Part model, mm, in its own coordinate system. Face numbers are marked on the shaded views. A direction names the side the tool comes from. Coordinates: 2 decimals unless noted, no trailing zeros. Order: outer loops, then holes, each group sorted by start corner. A loop starts at its lowest first (then second) coordinate and runs counter-clockwise, first axis right, second up.
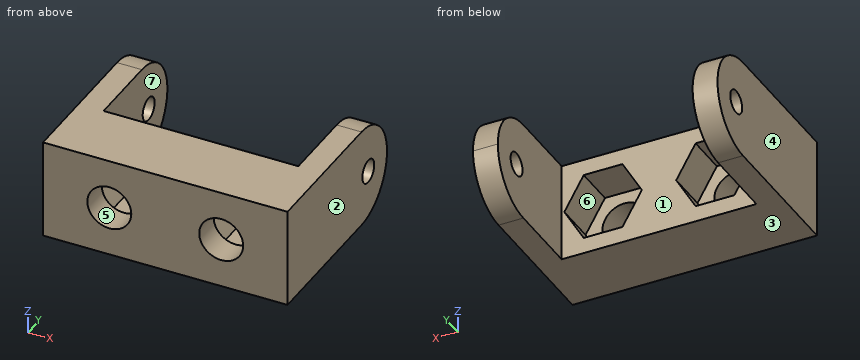
```python
from build123d import *

# Parameters (mm, degrees)
SKETCH_1_W          = 29.5
SKETCH_1_H          = 12
EXTRUDE_1_DEPTH     = 23.4
SKETCH_3_W          = 23.5
SKETCH_3_H          = 12
CUT_EXTRUDE_1_DEPTH = 15
SKETCH_4_R          = 1.4
CUT_EXTRUDE_2_DEPTH = 39.12886046
FILLET_1_RADIUS     = 6
FILLET_1_LENGTH     = 3
MIRROR_START        = 11.75
MIRROR_1_DEPTH      = 3
HOLE_WIZARD_M5_1_D  = 5.3
CUT_EXTRUDE_4_DEPTH = 5


# Read off the part's stored shape, not the designer's step: 镜向1
with BuildPart() as part:
    # 草图1 → 凸台-拉伸1 (new body)
    with BuildSketch(Plane(origin=(0, 0, 0), x_dir=(1, 0, 0), z_dir=(0, 1, 0))):
        Rectangle(SKETCH_1_W, SKETCH_1_H)
    extrude(amount=EXTRUDE_1_DEPTH)

    # 草图3 → 切除-拉伸1 (cut)
    with BuildSketch(Plane(origin=(0, 23.4, 0), x_dir=(1, 0, 0), z_dir=(0, 1, 0))):
        Rectangle(SKETCH_3_W, SKETCH_3_H)
    extrude(amount=-CUT_EXTRUDE_1_DEPTH, mode=Mode.SUBTRACT)

    # 草图4 → 切除-拉伸2 (cut, through all)
    with BuildSketch(Plane.ZY.offset(14.75)):
        with Locations((0, 19)):
            Circle(SKETCH_4_R)
    extrude(amount=-CUT_EXTRUDE_2_DEPTH, mode=Mode.SUBTRACT)

    # 圆角1: full round fillet: the end face becomes a half cylinder, R = half its width
    fillet_1_face = Plane((-13.25, 23.4, 0), x_dir=(-1, 0, 0), z_dir=(0, 1, 0))  # on the end face: x along it, z out of the body
    fillet_1_slab = fillet_1_face.offset(-FILLET_1_RADIUS / 2) * Box(FILLET_1_LENGTH, 2 * FILLET_1_RADIUS, FILLET_1_RADIUS, mode=Mode.PRIVATE)  # the body's end, R deep
    fillet_1_round = Plane((-13.25, 17.4, 0), x_dir=(0, 1, 0), z_dir=(-1, 0, 0)) * Cylinder(FILLET_1_RADIUS, FILLET_1_LENGTH, mode=Mode.PRIVATE)  # its axis R under the face
    add(fillet_1_slab - fillet_1_round, mode=Mode.SUBTRACT)

    # 镜向1 outline → 镜向1 (cut)
    with BuildSketch(Plane.YZ.offset(MIRROR_START)):
        with BuildLine():
            Line((23.4, 6), (17.4, 6))
            ThreePointArc((17.4, 6), (21.642640687, 4.242640687), (23.4, 0))
            Line((23.4, 0), (23.4, 6))
        make_face()
        with BuildLine():
            Line((23.4, -6), (23.4, 0))
            ThreePointArc((23.4, 0), (21.642640687, -4.242640687), (17.4, -6))
            Line((17.4, -6), (23.4, -6))
        make_face()
    extrude(amount=MIRROR_1_DEPTH, mode=Mode.SUBTRACT)

    # M5 间隙孔1 (through all)
    with Locations(Plane(origin=(0, 0, 0), x_dir=(-1, 0, 0), z_dir=(0, -1, 0))):
        with Locations((-6.75, 0), (6.75, 0)):
            Hole(HOLE_WIZARD_M5_1_D / 2)

    # 草图10 → 切除-拉伸4 (cut)
    with BuildSketch(Plane.XZ.offset(-8.4)):
        Polygon((2.07346282, 0), (4.41173141, -4.05), (9.08826859, -4.05), (11.42653718, 0), (9.08826859, 4.05), (4.41173141, 4.05), align=None)
        Polygon((-11.42653718, 0), (-9.08826859, -4.05), (-4.41173141, -4.05), (-2.07346282, 0), (-4.41173141, 4.05), (-9.08826859, 4.05), align=None)
    extrude(amount=CUT_EXTRUDE_4_DEPTH, mode=Mode.SUBTRACT)


solid = part.part
```
(1) Pull direction X, two halves, no side cores. Call the marked faces 1, 2, 3 and 4: +X half, -X half, draft (parallel to the pull), parting line (faces both ways), or undercut.
(2) Drop flat-ended pins along their axis: pin 1 (6.5 mm diameter, centred on x = -5.5, z = -2, fed in from +Y); pin 2 (3 mm diameter, centred on x = 6.75, z = 0, fed in from -Y); pin 3 (6 mm diameter, centred on x = -6.75, z = 0, fed in from +Y). Give the stop position or say it passes through.
(3) Probe line 1 (X direction, y = 7.5, z = 3.5); line 2 (X direction, y = 13.25, z = 2); line 3 (X direction, y = 1.25, z = -1.5). List the from-to ranges inside material, lowest first.
(4) Slice it at B-B, the plane x = 6.75. Give the cut face in (y, z), then the cut area to 3 significant figures.
(5) Slice it at C-C, the plane z = -1.75. Give the cut face in (x, y), then the cut area to 3 significant figures.
(6) Tool access for the marked faces 5, 6 and 7: list every direction of +Z, -Z, +X, -X, +Y, -Y with a clear straight run to the whole face (end or side of a thin tool).
(7) Slice it at A-A, the plane y = 11. Give the cut face in (x, z).
(8) Slice it at D-D, the plane y = 8. Give the cut face in (x, z), then the cut area to 3 significant figures.
Here are the results:
1. face 1: undercut
1. face 2: +X half
1. face 3: draft
1. face 4: -X half
2. pin 1: stops at y = 8.4
2. pin 2: passes through
2. pin 3: stops at y = 3.4
3. line 1: x = -14.75 to -9.41, -4.09 to 4.09, 9.41 to 14.75
3. line 2: x = -14.75 to -11.75, 11.75 to 14.75
3. line 3: x = -14.75 to -8.93, -4.57 to 4.57, 8.93 to 14.75
4. outline: (0, -6) - (8.4, -6) - (8.4, -4.05) - (3.4, -4.05) - (3.4, -2.65) - (0, -2.65) - close; (0, 2.65) - (3.4, 2.65) - (3.4, 4.05) - (8.4, 4.05) - (8.4, 6) - (0, 6) - close
4. area: 42.3 mm2
5. outline: (-14.75, 0) - (-8.74, 0) - (-8.74, 3.4) - (-10.42, 3.4) - (-10.42, 8.4) - (-11.75, 8.4) - (-11.75, 23.14) - (-14.75, 23.14) - close; (-4.76, 0) - (4.76, 0) - (4.76, 3.4) - (3.08, 3.4) - (3.08, 8.4) - (-3.08, 8.4) - (-3.08, 3.4) - (-4.76, 3.4) - close; (8.74, 0) - (14.75, 0) - (14.75, 23.14) - (11.75, 23.14) - (11.75, 8.4) - (10.42, 8.4) - (10.42, 3.4) - (8.74, 3.4) - close
5. area: 236 mm2
6. face 5: +Y, -Y
6. face 6: +Y
6. face 7: +Z, -Z, +Y
7. outline: (-14.75, -6) - (-11.75, -6) - (-11.75, 6) - (-14.75, 6) - close; (11.75, -6) - (14.75, -6) - (14.75, 6) - (11.75, 6) - close
8. outline: (-14.75, -6) - (14.75, -6) - (14.75, 6) - (-14.75, 6) - close; hole (-11.43, 0) - (-9.09, -4.05) - (-4.41, -4.05) - (-2.07, 0) - (-4.41, 4.05) - (-9.09, 4.05) - close; hole (2.07, 0) - (4.41, -4.05) - (9.09, -4.05) - (11.43, 0) - (9.09, 4.05) - (4.41, 4.05) - close
8. area: 240 mm2
